```python
from build123d import *

# Parameters (mm, degrees)
SKETCH1_R           = 18
SKETCH1_R_2         = 1.5
SKETCH1_R_3         = 4.2
BOSS_EXTRUDE2_DEPTH = 20.73


with BuildPart() as part:
    # Sketch1 → Boss-Extrude2 (new body)
    with BuildSketch(Plane.XY):
        Circle(SKETCH1_R)
        with Locations((0, 10)):
            Circle(SKETCH1_R_2, mode=Mode.SUBTRACT)
        Circle(SKETCH1_R_3, mode=Mode.SUBTRACT)
        with Locations((10, 0)):
            Circle(SKETCH1_R_2, mode=Mode.SUBTRACT)
        with Locations((0, -10)):
            Circle(SKETCH1_R_2, mode=Mode.SUBTRACT)
        with Locations((-10, 0)):
            Circle(SKETCH1_R_2, mode=Mode.SUBTRACT)
    extrude(amount=BOSS_EXTRUDE2_DEPTH)


solid = part.part
```
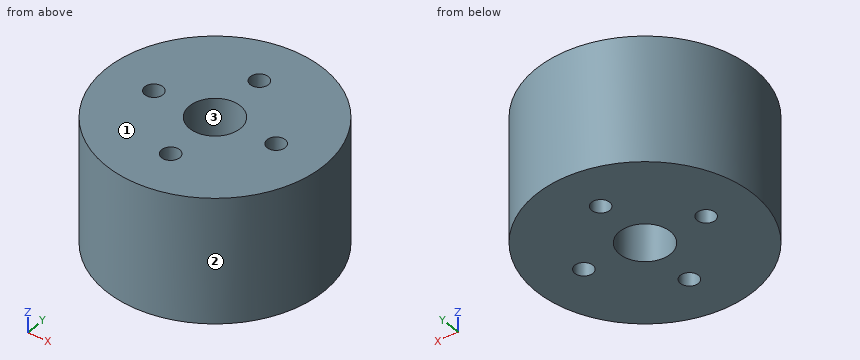
Verification items for the finished model (mm, model axes). Face numbers are marked on the shaded views. Coordinates: 2 decimals unless noted, no trailing zeros. Order: outer loops, then holes, each group sorted by start corner. A loop starts at its lowest first (then second) coordinate and runs counter-clockwise, first axis right, second up. Notation, with made-up numbers: (-14.5, -28) - (21.5, -28) arc R16 ccw to (21.5, -5) - close; hole circle Ø7 at (55, 58). An arc over 180 degrees is marked (long way). Return JSON: item names as keys, results as strings.
(1) Go/stop test with flat-tipped pins: pin 1 (6 mm diameter, centred on y = 8.5, z = 5, fed in from -X); pin 2 (2 mm diameter, centred on y = 10.5, z = 10.5, fed in from -X); pin 3 (1.5 mm diameter, centred on y = 9.5, z = 7.5, fed in from +X). Record where each tip stops, or that it passes through.
Filled sheet:
{"pin 1": "stops at x = -17.14", "pin 2": "stops at x = -15.29", "pin 3": "stops at x = 15.73"}
(2) Section check C-C, the plane z = 4.5. Record the cut outline in (x, y), and give its area (3 significant figures).
Filled sheet:
{"outline": "circle Ø36 at (0, 0); hole circle Ø3 at (-10, 0); hole circle Ø8.4 at (0, 0); hole circle Ø3 at (0, -10); hole circle Ø3 at (0, 10); hole circle Ø3 at (10, 0)", "area": "934 mm^2"}
(3) Section check A-A, the plane y = 0. Record the cut outline in (x, z), and give its area (3 significant figures).
Filled sheet:
{"outline": "(-18, 0) - (-11.5, 0) - (-11.5, 20.73) - (-18, 20.73) - close; (-8.5, 0) - (-4.2, 0) - (-4.2, 20.73) - (-8.5, 20.73) - close; (4.2, 0) - (8.5, 0) - (8.5, 20.73) - (4.2, 20.73) - close; (11.5, 0) - (18, 0) - (18, 20.73) - (11.5, 20.73) - close", "area": "448 mm^2"}
(4) Mould release check, pull along Y, two halves, no side actions. Record for the marked faces 1, 2 and 3: pulls with the +Y half, pulls with the -Y half, needs draft (parallel to the pull), parting line crosses it, or undercut.
Filled sheet:
{"face 1": "needs draft", "face 2": "parting line crosses it", "face 3": "undercut"}
(5) Thickness scan on line 1 along Y through (x, z) = (0, 10.25); line 2 along X through (y, z) = (1, 5.75); line 3 along Y through (x, z) = (9.5, 9.25). Record the ranges inside material, lowest first.
Filled sheet:
{"line 1": "y = -18 to -11.5, -8.5 to -4.2, 4.2 to 8.5, 11.5 to 18", "line 2": "x = -17.97 to -11.12, -8.88 to -4.08, 4.08 to 8.88, 11.12 to 17.97", "line 3": "y = -15.29 to -1.41, 1.41 to 15.29"}
(6) Section check B-B, the plane x = -10. Record the cut outline in (y, z), and give its area (3 significant figures).
Filled sheet:
{"outline": "(-14.97, 0) - (-1.5, 0) - (-1.5, 20.73) - (-14.97, 20.73) - close; (1.5, 0) - (14.97, 0) - (14.97, 20.73) - (1.5, 20.73) - close", "area": "558 mm^2"}
